Check sheet for the modelled part. Datum: model origin and axes. Units: mm. A direction names the side the tool comes from. Give positions to 0.01 mm unless a question says otherwise; leave off trailing zeros. Write each loop counter-clockwise with the first axis right and the second up, starting at its lowest first coordinate (ties: lowest second). Pieces come first, ordered by that corner, then holes. Notation, with made-up numbers: (30.5, -6.75) -> (35.5, -6.75) arc R26 cw to (35.5, 19.25) -> close; hole circle Ø4 at (56, 76.5). An arc over 180 degrees is marked (long way). Write each question's results on one line, items separated by ' | '. Start each with the question number.
```python
from build123d import *

# Parameters (mm, degrees)
F0_W     = 47.5
F0_H     = 47.5
F1_DEPTH = 1.6
F2_W     = 9
F2_H     = 14
F3_DEPTH = 12.54
F2_W_2   = 8
F2_H_2   = 10.806212
F4_DEPTH = 5.54
F2_R     = 0.815
F5_DEPTH = 1.6


with BuildPart() as f1:
    # F0 (on Top) → F1 (new body)
    with BuildSketch(Plane.XY):
        Rectangle(F0_W, F0_H)
    extrude(amount=F1_DEPTH)

    # F2 (on face) → F3 (join)
    with BuildSketch(Plane.XY.offset(1.6)):
        with Locations((9.25, -16.75)):
            Rectangle(F2_W, F2_H)
    extrude(amount=F3_DEPTH)

    # F2 (on face) → F4 (join)
    with BuildSketch(Plane.XY.offset(1.6)):
        with Locations((11.95, 18.346894)):
            Rectangle(F2_W_2, F2_H_2)
    extrude(amount=F4_DEPTH)

    # F2 (on face) → F5 (cut)
    with BuildSketch(Plane.XY.offset(1.6)):
        with Locations((-22.53, -22.53)):
            Circle(F2_R)
        with Locations((22.53, -22.53)):
            Circle(F2_R)
        with Locations((22.53, 22.53)):
            Circle(F2_R)
        with BuildLine():
            ThreePointArc((-21.715, 22.53), (-22.216277, 23.282199), (-23.103473, 23.109097))
            ThreePointArc((-23.103473, 23.109097), (-22.843723, 21.777801), (-21.715, 22.53))
        make_face()
    extrude(amount=-F5_DEPTH, mode=Mode.SUBTRACT)


solid = f1.part
```
Item 1: Depth check by flat-ended pin: pin 1 Ø1.3 at (x, y) = (22.53, -22.53) entering from -Z; pin 2 Ø3 at (y, z) = (20.5, 3.5) entering from -X; pin 3 Ø6.5 at (y, z) = (-14.5, 8.5) entering from +X; pin 4 Ø1.9 at (x, y) = (-22.53, -22.53) entering from +Z. Enter the tip coordinate at first touch or a pass-through.
Item 2: Section check B-B on x = -22.53. Record the boundary of the cut face in (y, z) (3 decimals), then the cut area to 3 significant figures.
Item 3: Section check A-A on z = 2.5. Record the boundary of the cut face in (x, y), then the cut area to 3 significant figures.
Item 4: Thickness scan on probe 1 along Y at (x, z) = (22.53, 1.25) (3 decimals); probe 2 along Z at (x, y) = (7.5, 8); probe 3 along Y at (x, z) = (7, 12.5). Record the ranges inside material, lowest first. Write a range as from..to.
Item 5: Mould release check, pull along X, two halves, no side actions. Record for faces 1 (the flat face through (-23.75, 0, 1)), 2 (the flat face through (13.75, -17, 8)), 3 (the flat face through (9, -17, 14.14)), 4 (the cylindrical face through (22.424, 23.338, 0.811)): pulls with the +X half, pulls with the -X half, needs draft (parallel to the pull), parting line crosses it, or undercut.
Item 6: Set-up check for faces 5 (the flat face through (15.95, 18, 4)), 6 (the flat face through (7.95, 18, 4)), 7 (the flat face through (4.75, -17, 8)), 8 (the flat face through (12, 18, 7.14)): record each of +Z, -Z, +X, -X, +Y, -Y from which the full face is reachable in a straight line by a thin tool's end or side.
Item 7: Section check D-D on y = 16.5. Record the boundary of the cut face in (x, z).
Item 8: Section check C-C on y = -22.53. Record the boundary of the cut face in (x, z) (3 decimals).
Check sheet entries:
1) pin 1: passes through | pin 2: stops at x = 7.95 | pin 3: stops at x = 13.75 | pin 4: stops at z = 1.6
2) outline: (-23.75, 0) -> (-23.345, 0) -> (-23.345, 1.6) -> (-23.75, 1.6) -> close; (-21.715, 0) -> (21.715, 0) -> (21.715, 1.6) -> (-21.715, 1.6) -> close; (23.345, 0) -> (23.75, 0) -> (23.75, 1.6) -> (23.345, 1.6) -> close | area: 70.8 mm^2
3) outline: (4.75, -23.75) -> (13.75, -23.75) -> (13.75, -9.75) -> (4.75, -9.75) -> close; (7.95, 12.94) -> (15.95, 12.94) -> (15.95, 23.75) -> (7.95, 23.75) -> close | area: 212 mm^2
4) probe 1: y = -23.75..-23.345, -21.715..21.715, 23.345..23.75 | probe 2: z = 0..1.6 | probe 3: y = -23.75..-9.75
5) face 1: pulls with the -X half | face 2: pulls with the +X half | face 3: needs draft | face 4: undercut
6) face 5: +Z, +X, +Y, -Y | face 6: +Z, -X, +Y | face 7: +Z, -X, +Y, -Y | face 8: +Z, +X, -X, +Y
7) outline: (-23.75, 0) -> (23.75, 0) -> (23.75, 1.6) -> (15.95, 1.6) -> (15.95, 7.14) -> (7.95, 7.14) -> (7.95, 1.6) -> (-23.75, 1.6) -> close
8) outline: (-23.75, 0) -> (-23.345, 0) -> (-23.345, 1.6) -> (-23.75, 1.6) -> close; (-21.715, 0) -> (21.715, 0) -> (21.715, 1.6) -> (13.75, 1.6) -> (13.75, 14.14) -> (4.75, 14.14) -> (4.75, 1.6) -> (-21.715, 1.6) -> close; (23.345, 0) -> (23.75, 0) -> (23.75, 1.6) -> (23.345, 1.6) -> close
